Autodesk Inventor part; units mm, degrees
ref_plane "YZ Plane" through (0, 0, 0) normal (1, 0, 0) x (0, 1, 0)
ref_plane "XZ Plane" through (0, 0, 0) normal (0, 1, 0) x (-1, 0, 0)
ref_plane "XY Plane" through (0, 0, 0) normal (0, 0, 1) x (1, 0, 0)
sketch "Sketch1" plane through (0, 0, 0) normal (0, 1, 0) x (-1, 0, 0)
  line L0 (15.6, 7) -> (-15.6, 7)
  line L1 (-15.6, 7) -> (-15.6, -7)
  line L2 (-15.6, -7) -> (15.6, -7)
  line L3 (15.6, -7) -> (15.6, 7)
  line L4 (15.6, 7) -> (-15.6, -7) construction
  line L5 (-15.6, 7) -> (15.6, -7) construction
  point P0 (0, 0)
  dimension "d0" = 31.2
  dimension "d1" = 14
extrude "Extrusion1" add sketch "Sketch1" along normal blind 1.5
sketch "Sketch2" plane through (0, 1.5, 0) normal (0, 1, 0) x (1, 0, 0)
  line L0 (9.1, -6.5) -> (15.1, -6.5)
  line L1 (15.1, -6.5) -> (15.1, 6.5)
  line L2 (15.1, 6.5) -> (9.1, 6.5)
  line L3 (9.1, 6.5) -> (9.1, -6.5)
  line L4 (9.1, -6.5) -> (15.1, 6.5) construction
  line L5 (15.1, -6.5) -> (9.1, 6.5) construction
  line L6 (15.6, 7) -> (-15.6, 7)
  line L7 (15.6, -7) -> (15.6, 7)
  point P0 (0, 0)
  point P1 (12.1, 0)
  point P2 (15.1, 0)
  point P3 (15.1, 0)
  dimension "d4" = 6
  dimension "d5" = 13
  dimension "d6" = 7
  dimension "d7" = 0.5
extrude "Extrusion2" add sketch "Sketch2" along normal blind 8
sketch "Sketch3" plane through (0, 9.5, 0) normal (0, 1, 0) x (1, 0, 0)
  line L0 (15.1, -6.5) -> (15.1, 6.5) construction
  line L1 (15.1, 6.5) -> (9.1, 6.5) construction
  line L2 (9.1, 6.5) -> (9.1, -6.5) construction
  line L3 (9.1, -6.5) -> (15.1, -6.5) construction
  line L4 (9.1, -6.5) -> (15.1, -6.5)
  line L5 (15.1, -6.5) -> (15.1, -2.5)
  line L6 (15.1, -2.5) -> (9.1, -2.5)
  line L7 (9.1, -2.5) -> (9.1, -6.5)
  line L8 (9.1, 6.5) -> (15.1, 6.5)
  line L9 (15.1, 6.5) -> (15.1, 2.5)
  line L10 (15.1, 2.5) -> (9.1, 2.5)
  line L11 (9.1, 2.5) -> (9.1, 6.5)
  line L12 (9.1, -2.5) -> (15.1, -2.5)
  line L13 (15.1, -2.5) -> (15.1, 2.5)
  line L14 (15.1, 2.5) -> (9.1, 2.5)
  line L15 (9.1, 2.5) -> (9.1, -2.5)
  point P0 (0, 0)
  dimension "d10" = 4
  dimension "d11" = 4
extrude "Extrusion3" cut sketch "Sketch3" against normal blind 7 contours L15 L10 L13 L6
sketch "Sketch4" plane through (0, 1.5, 0) normal (0, 1, 0) x (1, 0, 0)
  line L0 (-15.6, 7) -> (-15.6, -7) construction
  line L1 (-15.6, 0) -> (-9.1, 0) construction
  point P0 (0, 0)
  dimension "d14" = 6.5
hole "Hole1" at (-9.1, 1.5, 0) direction (0, -1, 0) diameter 3.5 end through all
sketch "Sketch5" plane through (0, 1.5, 0) normal (0, 1, 0) x (1, 0, 0)
  circle A0 centre (-9.1, 0) radius 1.75 construction
  line L0 (15.1, -6.5) -> (9.1, -6.5) construction
  line L1 (9.1, -6.5) -> (9.1, 6.5) construction
  line L2 (9.1, 6.5) -> (15.1, 6.5) construction
  line L3 (15.1, 6.5) -> (15.1, -6.5) construction
  line L4 (15.6, -7) -> (15.6, 7) construction
  line L5 (15.6, 7) -> (-15.6, 7) construction
  line L6 (-15.6, 7) -> (-15.6, -7) construction
  line L7 (-15.6, -7) -> (15.6, -7) construction
  line L8 (-23.6, 4.5) -> (-13.6, 4.5)
  line L9 (-13.6, 4.5) -> (-13.6, -4.5)
  line L10 (-13.6, -4.5) -> (-23.6, -4.5)
  line L11 (-23.6, -4.5) -> (-23.6, 4.5)
  line L12 (-13.6, 7) -> (-13.6, -7) construction
  point P0 (0, 0)
  point P1 (-13.6, 0)
  dimension "d22" = 10
  dimension "d23" = 9
  dimension "d24" = 2
extrude "Extrusion4" add sketch "Sketch5" along normal blind 4
properties part number "irencoder_footprint"
Input: part model. Units: mm. Frame: model coordinates. A direction names the side the tool comes from. Round coordinates to 2 decimals unless told otherwise and drop trailing zeros. Order: outer loops, then holes, each group sorted by start corner. A loop starts at its lowest first (then second) coordinate and runs counter-clockwise, first axis right, second up. Notation, with made-up numbers: (5.5, 52.25) - (48.5, 52.25) arc R17 ccw to (48.5, 59.25) - close; hole circle Ø8 at (51, 69.5). An arc over 180 degrees is marked (long way). Use a Markdown table: item, result.
1. Material intervals for probe 1 along Z at (x, y) = (-9.1, 0.75); probe 2 along X at (y, z) = (0.9, 0); probe 3 along Y at (x, z) = (-19.5, -1.5), sorted ascending.
Evaluation:
| item | result |
|---|---|
| probe 1 | -7 to -1.75, 1.75 to 7 |
| probe 2 | -15.6 to -10.85, -7.35 to 15.6 |
| probe 3 | 1.5 to 5.5 |
2. Section C-C on z = 0. Return the cut outline in (x, y), then the cut area to 4 significant figures.
Evaluation:
| item | result |
|---|---|
| outline | (-23.6, 1.5) - (-15.6, 1.5) - (-15.6, 0) - (-10.85, 0) - (-10.85, 1.5) - (-13.6, 1.5) - (-13.6, 5.5) - (-23.6, 5.5) - close; (-7.35, 0) - (15.6, 0) - (15.6, 1.5) - (15.1, 1.5) - (15.1, 2.5) - (9.1, 2.5) - (9.1, 1.5) - (-7.35, 1.5) - close |
| area | 87.55 mm^2 |
3. Section D-D on y = 8.25. Return the cut outline in (x, z).
Evaluation:
| item | result |
|---|---|
| outline | (9.1, -6.5) - (15.1, -6.5) - (15.1, -2.5) - (9.1, -2.5) - close; (9.1, 2.5) - (15.1, 2.5) - (15.1, 6.5) - (9.1, 6.5) - close |
4. First-contact query: pin 1 (4 mm diameter, centred on y = 5.5, z = 2.5, fed in from +X); pin 2 (1.8 mm diameter, centred on x = 12, y = 7.5, fed in from -Z); pin 3 (1.5 mm diameter, centred on x = 11.5, z = 1, fed in from +Y). Flat tips, straight axial feed; report the tip coordinate or a pass-through.
Evaluation:
| item | result |
|---|---|
| pin 1 | x = 15.1 |
| pin 2 | z = -6.5 |
| pin 3 | y = 2.5 |
5. Mould query, pull axis X, two halves, no side actions, for faces 5 (the face through (-13.6, 3, 0)), 6 (the face through (-23.6, 3, 0)), 7 (the face through (15.1, 5, 3)), 8 (the face through (0, 1, 7)). Classes: +X half, -X half, draft (parallel to the pull), parting line (faces both ways), or undercut.
Evaluation:
| item | result |
|---|---|
| face 5 | undercut |
| face 6 | -X half |
| face 7 | +X half |
| face 8 | draft |
6. Section A-A on y = 4.75. Return the cut outline in (x, z), then the cut area to 3 significant figures.
Evaluation:
| item | result |
|---|---|
| outline | (-23.6, -4.5) - (-13.6, -4.5) - (-13.6, 4.5) - (-23.6, 4.5) - close; (9.1, -6.5) - (15.1, -6.5) - (15.1, -2.5) - (9.1, -2.5) - close; (9.1, 2.5) - (15.1, 2.5) - (15.1, 6.5) - (9.1, 6.5) - close |
| area | 138 mm^2 |
7. Access query for faces 1 (the face through (-19, 5.5, 0)), 2 (the face through (12, 6, 2.5)), 3 (the face through (-19, 3, -4.5)), 4 (the face through (-15.6, 1, 0)). Directions: +Z, -Z, +X, -X, +Y, -Y. A direction counts if a zero-diameter tool reaches every point of the face in a straight line with its end or side. Return the directions, or none.
Evaluation:
| item | result |
|---|---|
| face 1 | +Z, -Z, -X, +Y |
| face 2 | +X, +Y |
| face 3 | -Z, -X, +Y |
| face 4 | +Z, -Z, -X, -Y |
8. Section B-B on x = -9.1. Return the cut outline in (y, z), then the cut area to 4 significant figures.
Evaluation:
| item | result |
|---|---|
| outline | (0, -7) - (1.5, -7) - (1.5, -1.75) - (0, -1.75) - close; (0, 1.75) - (1.5, 1.75) - (1.5, 7) - (0, 7) - close |
| area | 15.75 mm^2 |
